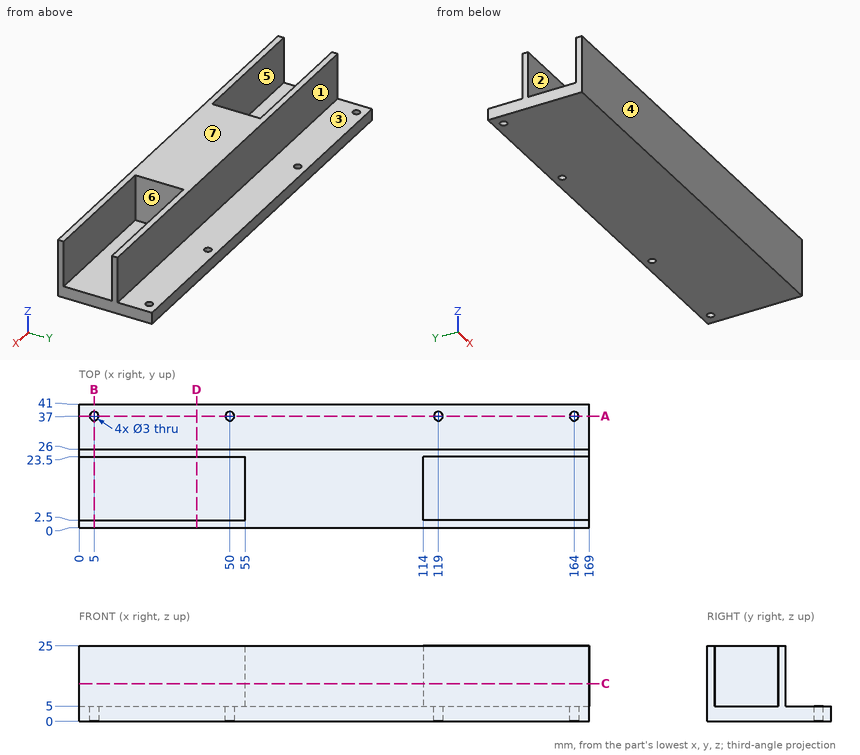
Source: three-view drawing plus pictorial views. Frame: mm from the lowest corner of the part. A direction names the side the tool comes from. Round coordinates to 2 decimals unless told otherwise and drop trailing zeros. Write each loop counter-clockwise with the first axis right and the second up, starting at its lowest first coordinate (ties: lowest second). Pieces come first, ordered by that corner, then holes. Notation, with made-up numbers: M 83,-38 L 108,-38 A20 ccw 108,-2 Z; hole C -23,63.25 d3. An arc over 180 degrees is marked long. Write each question's results on one line, items separated by ' | '.
Q1. Section query C-C (z = 12.5). Return loops of the section in (x, y), and give its area (3 significant figures).
Results:
outline: M 0,0 L 169,0 L 169,2.5 L 114,2.5 L 114,23.5 L 169,23.5 L 169,26 L 0,26 L 0,23.5 L 55,23.5 L 55,2.5 L 0,2.5 Z | area: 2,080 mm^2
Q2. Pin query (flat end, axial travel): P1, Ø1.5, axis at x = 146, z = 16, coming from the +Y side; P2, Ø3, axis at y = 16, z = 3.5, coming from the -X side; P3, Ø16.5, axis at x = 76, y = 34.5, coming from the +Z side; P4, Ø1.5, axis at y = 22.5, z = 20.5, coming from the +X side. Return the tip coordinate at first contact, or that it passes through.
Results:
P1: stops at y = 26 | P2: stops at x = 0 | P3: stops at z = 5 | P4: stops at x = 114
Q3. Draft query along Y for the marked faces 1, 2, 3 and 4. Return one class per face: released by +Y, released by -Y, zero draft, split by the parting line, or undercut.
Results:
face 1: released by +Y | face 2: undercut | face 3: zero draft | face 4: released by -Y
Q4. Section query B-B (x = 5). Return loops of the section in (y, z).
Results:
outline: M 0,0 L 35.5,0 L 35.5,5 L 26,5 L 26,25 L 23.5,25 L 23.5,5 L 2.5,5 L 2.5,25 L 0,25 Z; M 38.5,0 L 41,0 L 41,5 L 38.5,5 Z
Q5. Section query D-D (x = 39). Return loops of the section in (y, z), and give its area (3 significant figures).
Results:
outline: M 0,0 L 41,0 L 41,5 L 26,5 L 26,25 L 23.5,25 L 23.5,5 L 2.5,5 L 2.5,25 L 0,25 Z | area: 305 mm^2
Q6. Access query for the marked faces 5, 6 and 7. Directions: +Z, -Z, +X, -X, +Y, -Y. A direction counts if a zero-diameter tool reaches every point of the face in a straight line with its end or side. Return the directions, or none.
Results:
face 5: +Z, -X | face 6: +Z, +X | face 7: +Z, +X, -X, +Y, -Y
Q7. Section query A-A (y = 37). Return loops of the section in (x, z), and give its area (3 significant figures).
Results:
outline: M 0,0 L 3.5,0 L 3.5,5 L 0,5 Z; M 6.5,0 L 48.5,0 L 48.5,5 L 6.5,5 Z; M 51.5,0 L 117.5,0 L 117.5,5 L 51.5,5 Z; M 120.5,0 L 162.5,0 L 162.5,5 L 120.5,5 Z; M 165.5,0 L 169,0 L 169,5 L 165.5,5 Z | area: 785 mm^2
Q8. Line query: line 1 along Y through (x, z) = (50, 1.2); line 2 along Y through (x, z) = (127.5, 14.75); line 3 along Y through (x, z) = (64, 10.5). Output: solid intervals per line, ascending.
Results:
line 1: y = 0 to 35.5, 38.5 to 41 | line 2: y = 0 to 2.5, 23.5 to 26 | line 3: y = 0 to 26
